```python
from build123d import *

# Parameters (mm, degrees)
BOSS_EXTRUDE1_DEPTH = 5
SKETCH2_R           = 13
CUT_EXTRUDE1_DEPTH  = 5


with BuildPart() as part:
    # Sketch1 → Boss-Extrude1 (new body)
    with BuildSketch(Plane(origin=(0, 0, 0), x_dir=(1, 0, 0), z_dir=(0, 1, 0))):
        with BuildLine():
            Line((248.032931618, 52.593341059), (260.305567907, 25.2785247))
            ThreePointArc((260.305567907, 25.2785247), (260.612237386, 17.847313664), (255.703480887, 12.259733394))
            Line((255.703480887, 12.259733394), (41.520626689, -96.255259938))
            ThreePointArc((41.520626689, -96.255259938), (37.001121909, -97.334829649), (32.481617129, -96.255259938))
            Line((32.481617129, -96.255259938), (-181.70123707, 12.259733394))
            ThreePointArc((-181.70123707, 12.259733394), (-186.609993569, 17.847313664), (-186.30332409, 25.2785247))
            Line((-186.30332409, 25.2785247), (-174.0306878, 52.593341059))
            Line((-174.0306878, 52.593341059), (248.032931618, 52.593341059))
        make_face()
    extrude(amount=BOSS_EXTRUDE1_DEPTH)

    # Sketch2 → Cut-Extrude1 (cut)
    with BuildSketch(Plane(origin=(0, 5, 0), x_dir=(1, 0, 0), z_dir=(0, 1, 0))):
        with Locations(Location((137.001121909, 12.593341059, 0), (0, 0, 270))):
            Circle(SKETCH2_R)
        with Locations(Location((-62.998878091, 12.593341059, 0), (0, 0, 270))):
            Circle(SKETCH2_R)
    extrude(amount=-CUT_EXTRUDE1_DEPTH, mode=Mode.SUBTRACT)


solid = part.part
```
The model under review builds one solid part; all positions refer to its coordinate system, in mm. Round coordinates to 2 decimals unless told otherwise and drop trailing zeros. Order: outer loops, then holes, each group sorted by start corner. A loop starts at its lowest first (then second) coordinate and runs counter-clockwise, first axis right, second up.
(1) Take a section at B-B, the plane z = -4.5. State the section outline as (x, y) points.
Working result:
outline: (-166.39, 0) - (-73.17, 0) - (-73.17, 5) - (-166.39, 5) - close; (-52.83, 0) - (126.83, 0) - (126.83, 5) - (-52.83, 5) - close; (147.17, 0) - (240.39, 0) - (240.39, 5) - (147.17, 5) - close
(2) Take a section at C-C, the plane x = 98.5. State the section outline as (y, z) points.
Working result:
outline: (0, -52.59) - (5, -52.59) - (5, 67.39) - (0, 67.39) - close
(3) Take a section at D-D, the plane z = 37. State the section outline as (x, y) points, plus the area to 3 significant figures.
Working result:
outline: (-84.47, 0) - (158.48, 0) - (158.48, 5) - (-84.47, 5) - close
area: 1,210 mm2
(4) Mouldability with a two-part tool opening along X and no side actions: class faces 1 (the face through (-50.11, 2.54, -14.29)), 2 (the face through (149.89, 2.54, -14.29)), 3 (the face through (40, 5, 5)), 4 (the face through (-73.111, 2.465, 42.757)) as released by +X, released by -X, zero draft, split by the parting line, or undercut.
Working result:
face 1: undercut
face 2: undercut
face 3: zero draft
face 4: released by -X
(5) Wall thickness on L1, parallel to X at y = 4, z = -15; L2, parallel to X at y = 4.6, z = -11; L3, parallel to X at y = 1.2, z = 24.5: over which ranges is each line inside the solid? List them lowest first.
Working result:
L1: x = -185.04 to -75.77, -50.22 to 124.23, 149.78 to 259.05
L2: x = -179.21 to -75.9, -50.1 to 124.1, 149.9 to 253.22
L3: x = -109.15 to 183.15
(6) For P1, Ø2, axis at y = 2, z = 50.5, coming from the +X side; P2, Ø3, axis at x = 53, z = 39.5, coming from the -Y side, all flat-tipped, find the tip position at first contact; note any pin that passes through.
Working result:
P1: stops at x = 133.8
P2: stops at y = 0
(7) Take a section at A-A, the plane y = 3.4. State the section outline as (x, z) points.
Working result:
outline: (-186.3, -25.28) - (-174.03, -52.59) - (248.03, -52.59) - (260.31, -25.28) arc R10 ccw to (255.7, -12.26) - (41.52, 96.26) arc R10 ccw to (32.48, 96.26) - (-181.7, -12.26) arc R10 ccw to start; hole circle Ø26 at (-63, -12.59); hole circle Ø26 at (137, -12.59)
